Design review of the part built by this model. Coordinates are the model's own, in mm. Face numbers are marked on the shaded views. A direction names the side the tool comes from. Round coordinates to 2 decimals unless told otherwise and drop trailing zeros. Order: outer loops, then holes, each group sorted by start corner. A loop starts at its lowest first (then second) coordinate and runs counter-clockwise, first axis right, second up. Notation, with made-up numbers: (88.25, -29) - (102.25, -29) arc R16 cw to (102.25, -2) - close; hole circle Ø8 at (21, 70.5). An arc over 180 degrees is marked (long way). Write item = value, one per line.
from build123d import *

# Parameters (mm, degrees)
BOSS_EXTRUDE1_DEPTH = 6.5


with BuildPart() as part:
    # Sketch1 → Boss-Extrude1 (new body)
    with BuildSketch(Plane(origin=(-63.134662924, 0, 0), x_dir=(0, 0, -1), z_dir=(1, 0, 0))):
        with BuildLine():
            Line((-10.565276343, -89.229749456), (-49.416189654, -60.285036457))
            ThreePointArc((-49.416189654, -60.285036457), (-61.41810481, -61.560228003), (-61.087779733, -73.625175837))
            Line((-61.087779733, -73.625175837), (-27.238976455, -108.287091427))
            ThreePointArc((-27.238976455, -108.287091427), (-8.594688607, -107.776631215), (-10.565276343, -89.229749456))
        make_face()
        with BuildLine():
            Line((-26.330356711, -107.399786428), (-60.179159989, -72.737870838))
            ThreePointArc((-60.179159989, -72.737870838), (-60.46229577, -62.39648698), (-50.174939921, -61.303465655))
            Line((-50.174939921, -61.303465655), (-46.502941226, -64.039178649))
            Line((-46.502941226, -64.039178649), (-11.32402661, -90.248178655))
            ThreePointArc((-11.32402661, -90.248178655), (-9.550497648, -106.940372237), (-26.330356711, -107.399786428))
        make_face(mode=Mode.SUBTRACT)
    extrude(amount=BOSS_EXTRUDE1_DEPTH)


solid = part.part
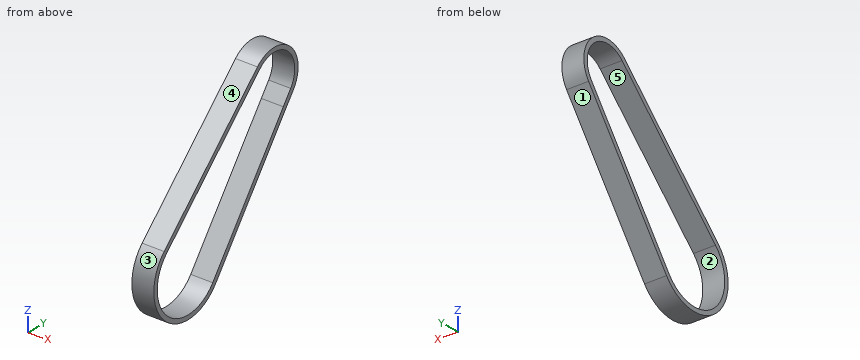
Item 1: Take a section at A-A, the plane x = -59.75. State the section outline as (y, z) points, and give its area (3 significant figures).
Data:
outline = (-108.29, 27.24) arc R12.7 ccw (long way) to (-89.23, 10.57) - (-60.29, 49.42) arc R8.89 ccw to (-73.63, 61.09) - close; hole (-107.4, 26.33) arc R11.43 ccw (long way) to (-90.25, 11.32) - (-61.3, 50.17) arc R7.62 ccw to (-72.74, 60.18) - close
area = 205 mm2
Item 2: The part is to be moulded in two halves that separate along Z. For the marked faces 1, 2 and 3, say which applies: +Z half, -Z half, draft (parallel to the pull), parting line (faces both ways), or undercut.
Data:
face_1 = -Z half
face_2 = undercut
face_3 = parting line
Item 3: For the marked faces 4 and 5, list the 3-axis set-ups (+Z, -Z, +X, -X, +Y, -Y) from which the entire face can be reached by the end or side of a thin tool; tool diameter is ignored.
Data:
face_4 = +Z, +X, -X, -Y
face_5 = +X, -X
Item 4: For line 1 along Z through (x, y) = (-63, -82.5); line 2 along Z through (x, y) = (-58, -60.5); line 3 along Y through (x, z) = (-62, 9.5), list the stretches that pass through material, from the lowest coordinate up. Write a range as [from, to].
Data:
line_1 = [19.6, 21.72], [50.65, 52.42]
line_2 = [49.13, 51.52], [57.93, 60.32]
line_3 = [-108.71, -106.88], [-91.95, -90.12]
Item 5: Insertion check: P1, Ø1.5, axis at x = -58.5, y = -88.5, coming from the -Z side; P2, Ø2, axis at x = -62, y = -74, coming from the +Z side; P3, Ø6, axis at y = -75.5, z = 31.5, coming from the -X side. Each pin has a flat end and moves straight along its axis. Give the tip position at first contact, or say it passes through.
Data:
P1 = 10.54
P2 = 61.64
P3 = -63.13
Item 6: Take a section at C-C, the plane z = 18. State the section outline as (x, y) points, and give its area (3 significant figures).
Data:
outline = (-63.13, -112.11) - (-56.63, -112.11) - (-56.63, -110.84) - (-63.13, -110.84) - close; (-63.13, -85.27) - (-56.63, -85.27) - (-56.63, -83.69) - (-63.13, -83.69) - close
area = 18.5 mm2
Item 7: Take a section at B-B, the plane y = -103.5. State the section outline as (x, z) points, and give its area (3 significant figures).
Data:
outline = (-63.13, 6.13) - (-56.63, 6.13) - (-56.63, 7.48) - (-63.13, 7.48) - close; (-63.13, 30.14) - (-56.63, 30.14) - (-56.63, 31.91) - (-63.13, 31.91) - close
area = 20.3 mm2
